Check sheet for the modelled part. Datum: model origin and axes. Units: mm. Coordinates: 2 decimals unless noted, no trailing zeros. Loops run counter-clockwise (first coordinate to the right, second up) from the corner with the lowest first, then second, coordinate; pieces in that order, holes last.
from build123d import *

# Parameters (mm, degrees)
BOSS_EXTRUDE1_DEPTH = 1.6
CUT_EXTRUDE1_DEPTH  = 10


with BuildPart() as part:
    # Sketch1 → Boss-Extrude1 (new body)
    with BuildSketch(Plane(origin=(0, 0, 0), x_dir=(1, 0, 0), z_dir=(0, 1, 0))):
        with BuildLine():
            Line((-24.15, 15.25), (-24.15, -15.25))
            Line((-24.15, -15.25), (-22.15, -15.25))
            Line((-22.15, -15.25), (-22.15, -20.967295963))
            ThreePointArc((-22.15, -20.967295963), (0, -30.5), (22.15, -20.967295963))
            Line((22.15, -20.967295963), (22.15, -15.25))
            Line((22.15, -15.25), (24.15, -15.25))
            Line((24.15, -15.25), (24.15, 15.25))
            Line((24.15, 15.25), (22.15, 15.25))
            Line((22.15, 15.25), (22.15, 20.967295963))
            ThreePointArc((22.15, 20.967295963), (0, 30.5), (-22.15, 20.967295963))
            Line((-22.15, 20.967295963), (-22.15, 15.25))
            Line((-22.15, 15.25), (-24.15, 15.25))
        make_face()
    extrude(amount=BOSS_EXTRUDE1_DEPTH)

    # Sketch2 → Cut-Extrude1 (cut)
    with BuildSketch(Plane(origin=(0, 1.6, 0), x_dir=(1, 0, 0), z_dir=(0, 1, 0))):
        with BuildLine():
            ThreePointArc((-10, 26.68801229), (0, 28.5), (10, 26.68801229))
            Line((10, 26.68801229), (10.701754386, 28.560855258))
            ThreePointArc((10.701754386, 28.560855258), (0, 30.5), (-10.701754386, 28.560855258))
            Line((-10.701754386, 28.560855258), (-10, 26.68801229))
        make_face()
    extrude(amount=-CUT_EXTRUDE1_DEPTH, mode=Mode.SUBTRACT)


solid = part.part
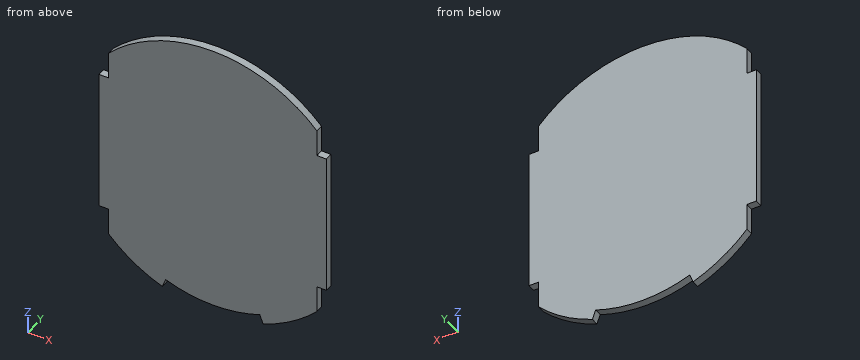
(1) Gauge pin test, flat ends, axial feed: P1, Ø0.5, axis at y = 0.5, z = -19, coming from the +X side; P2, Ø0.5, axis at x = -22.5, y = 0.5, coming from the +Z side; P3, Ø0.5, axis at x = -23, y = 1, coming from the -Z side. Record the tip position at first contact, or that the pin passes through.
(2) Section check A-A, the plane y = 0.3. Enter the section's corners in (x, z), plus the area to 3 significant figures.
(3) Section check B-B, the plane x = 17.5. Enter the section's corners in (y, z), plus the area to 3 significant figures.
(4) Scan lines: line 1 along X through (y, z) = (0.55, 16); line 2 along Z through (x, y) = (-0.5, 0.5); line 3 along Z through (x, y) = (-11, 0.25). Record each from-to range of solid material in increasing order.
(5) Section check C-C, the plane z = 22.5. Enter the section's corners in (x, y), plus the area to 3 significant figures.
Determined:
1. P1: stops at x = 22.15
1. P2: stops at z = 15.25
1. P3: stops at z = -15.25
2. outline: (-24.15, -15.25) - (-22.15, -15.25) - (-22.15, -20.97) arc R30.5 ccw to (-10.7, -28.56) - (-10, -26.69) arc R28.5 ccw to (10, -26.69) - (10.7, -28.56) arc R30.5 ccw to (22.15, -20.97) - (22.15, -15.25) - (24.15, -15.25) - (24.15, 15.25) - (22.15, 15.25) - (22.15, 20.97) arc R30.5 ccw to (-22.15, 20.97) - (-22.15, 15.25) - (-24.15, 15.25) - close
2. area: 2,520 mm2
3. outline: (0, -24.98) - (1.6, -24.98) - (1.6, 24.98) - (0, 24.98) - close
3. area: 79.9 mm2
4. line 1: x = -22.15 to 22.15
4. line 2: z = -28.5 to 30.5
4. line 3: z = -28.45 to 28.45
5. outline: (-20.59, 0) - (20.59, 0) - (20.59, 1.6) - (-20.59, 1.6) - close
5. area: 65.9 mm2
